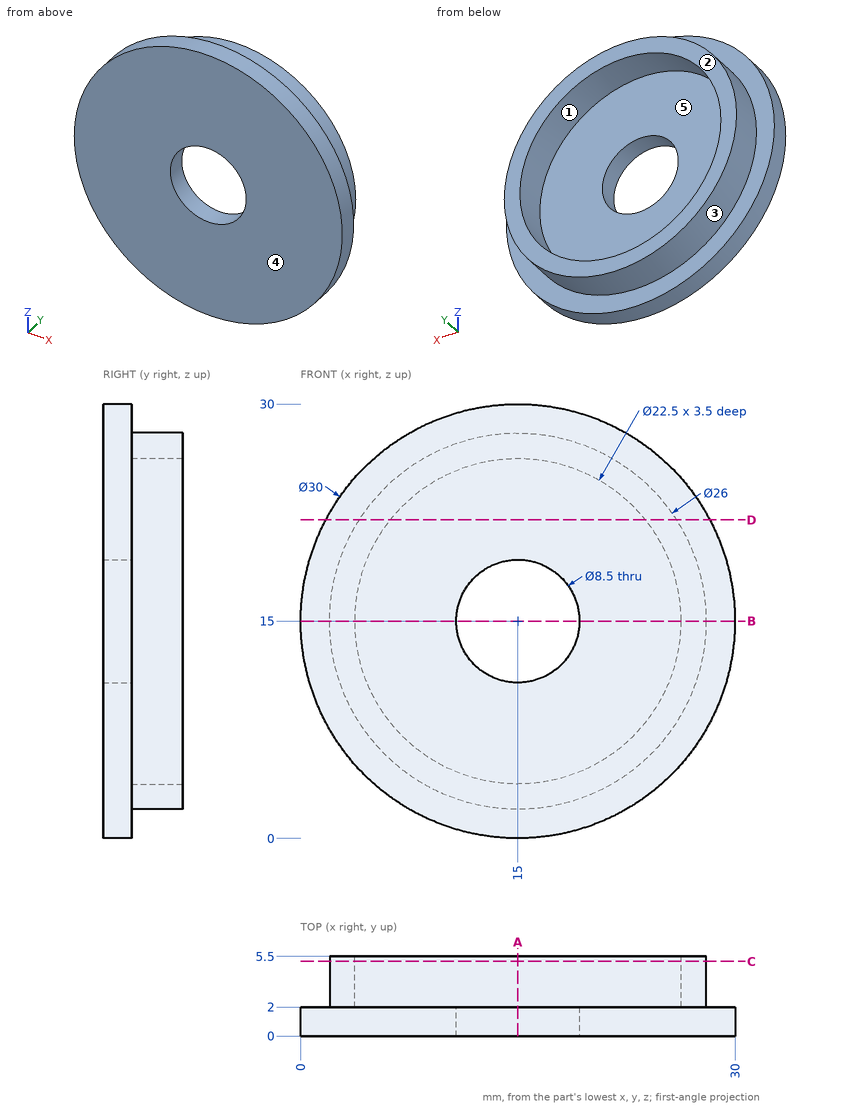
Design review of the part shown in the three views and the two pictorial views. Dimensions are in mm from the part's minimum x, y and z. A direction names the side the tool comes from. Give positions to 0.01 mm unless a question says otherwise; leave off trailing zeros. Loops run counter-clockwise (first coordinate to the right, second up) from the corner with the lowest first, then second, coordinate; pieces in that order, holes last. Notation, with made-up numbers: (89.25, 29) - (109.25, 29) arc R15 cw to (109.25, 41) - close; hole circle Ø7 at (80, -1). An arc over 180 degrees is marked (long way). Use CSV: the item, a comma, the result in double quotes. Start each with the question number.
1. Add section D-D (z = 22). State the section outline as (x, y) points, plus the area to 3 significant figures.
2. Insertion check: P1, Ø2, axis at x = 18.5, z = 22.5, coming from the +Y side; P2, Ø10, axis at x = 15, z = 15, coming from the -Y side; P3, Ø3, axis at x = 20.5, y = 2.5, coming from the -Z side. Each pin has a flat end and moves straight along its axis. Give the tip position at first contact, or say it passes through.
3. Machinability: for the marked faces 1 and 2, which of the approach directions +Z, -Z, +X, -X, +Y, -Y give a long, thin tool a straight path to every point of the face, cutting with its end or side? Answer none if there is none.
4. Add section A-A (x = 15). State the section outline as (y, z) points, plus the area to 4 significant figures.
5. Add section B-B (z = 15). State the section outline as (x, y) points.
6. Wall thickness on L1, parallel to Z at x = 15, y = 3.5; L2, parallel to Z at x = 15, y = 0.65; L3, parallel to Y at x = 25, z = 13.25: over which ranges is each line inside the solid? List them lowest first.
7. Draft analysis for pull direction X (two halves, no side actions). For the marked faces 3, 4 and 5, state which applies: released by +X, released by -X, zero draft, split by the parting line, or undercut.
8. Add section C-C (y = 5.15). State the section outline as (x, z) points, plus the area to 3 significant figures.
Results found:
1,outline,"(1.73, 0) - (28.27, 0) - (28.27, 2) - (25.95, 2) - (25.95, 5.5) - (23.81, 5.5) - (23.81, 2) - (6.19, 2) - (6.19, 5.5) - (4.05, 5.5) - (4.05, 2) - (1.73, 2) - close"
1,area,"68.1 mm²"
2,P1,"stops at y = 2"
2,P2,"stops at y = 0"
2,P3,"stops at z = 0.57"
3,face 1,"+Y"
3,face 2,"+Z, -Z, +X, -X, +Y"
4,outline,"(0, 0) - (2, 0) - (2, 2) - (5.5, 2) - (5.5, 3.75) - (2, 3.75) - (2, 10.75) - (0, 10.75) - close; (0, 19.25) - (2, 19.25) - (2, 26.25) - (5.5, 26.25) - (5.5, 28) - (2, 28) - (2, 30) - (0, 30) - close"
4,area,"55.25 mm²"
5,outline,"(0, 0) - (10.75, 0) - (10.75, 2) - (3.75, 2) - (3.75, 5.5) - (2, 5.5) - (2, 2) - (0, 2) - close; (19.25, 0) - (30, 0) - (30, 2) - (28, 2) - (28, 5.5) - (26.25, 5.5) - (26.25, 2) - (19.25, 2) - close"
6,L1,"z = 2 to 3.75, 26.25 to 28"
6,L2,"z = 0 to 10.75, 19.25 to 30"
6,L3,"y = 0 to 2"
7,face 3,"split by the parting line"
7,face 4,"zero draft"
7,face 5,"undercut"
8,outline,"circle Ø26 at (15, 15); hole circle Ø22.5 at (15, 15)"
8,area,"133 mm²"
